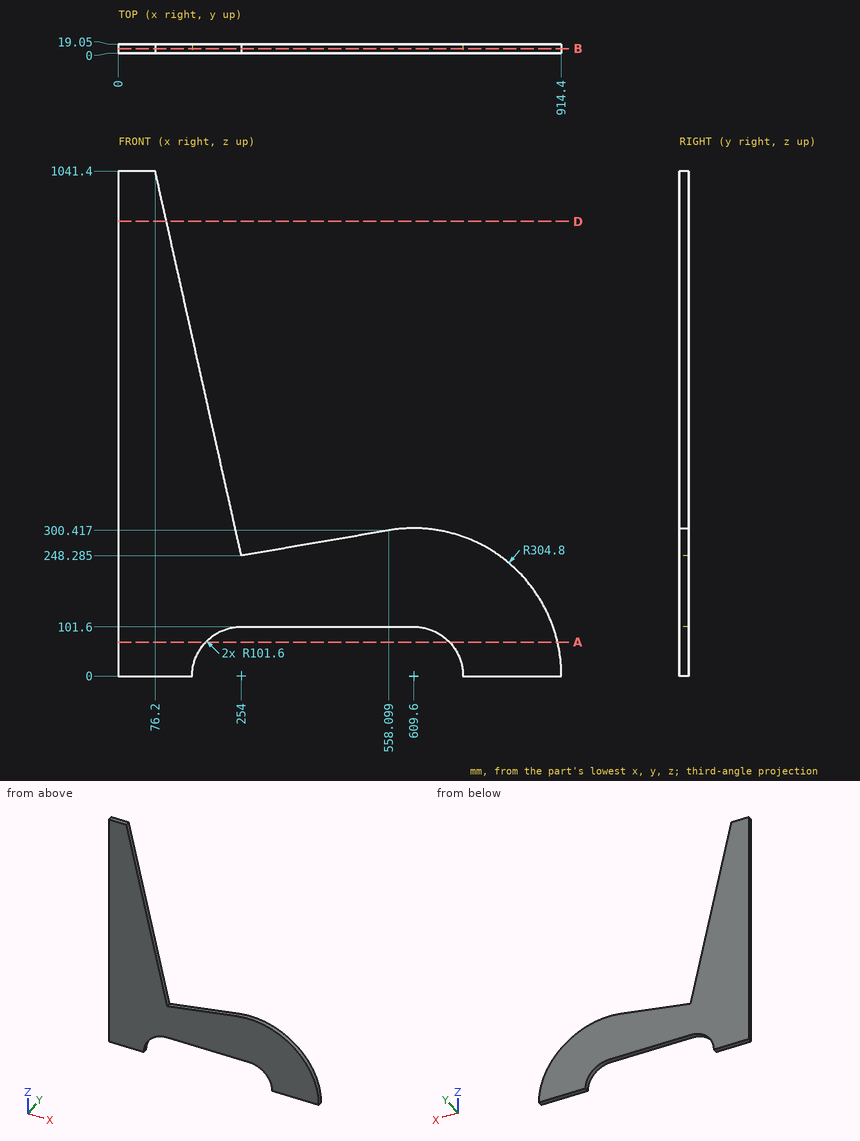
Print and shaded views of the part. All mm, measured from the part's lowest x, y and z. Coordinates: 2 decimals unless noted, no trailing zeros. Order: outer loops, then holes, each group sorted by start corner. A loop starts at its lowest first (then second) coordinate and runs counter-clockwise, first axis right, second up. Notation, with made-up numbers: M 28,-8 L 58,-8 A25 ccw 58,23 Z; hole C 87.5,-30 d9. An arc over 180 degrees is marked long. Write each question's results on one line, items separated by ' | '. Start each with the question number.
Q1. Cut at A-A (z = 70). List the corners of the cut face in (x, y).
Q2. Drill centre lines: probe 1 along X at (y, z) = (7.75, 856.5); probe 2 along X at (y, z) = (16.75, 963.5) (1 decimal); probe 3 along Z at (x, y) = (445, 17.5). Where is each one in solid material? Low to high. Write a range as from..to.
Q3. Cut at D-D (z = 938). List the corners of the cut face in (x, y).
Q4. Flat gauge pins, fed straight in: P1, Ø1.5, axis at y = 16.5, z = 257.5, coming from the +X side (1 decimal); P2, Ø10, axis at y = 4.5, z = 932, coming from the +X side; P3, Ø3, axis at x = 351, y = 11, coming from the +Z side. Where does each tip first touch, or does it go through?
Q5. Cut at B-B (y = 9.75). List the corners of the cut face in (x, z) (1 decimal).
Found:
1) outline: M 0,0 L 180.36,0 L 180.36,19.05 L 0,19.05 Z; M 683.24,0 L 906.25,0 L 906.25,19.05 L 683.24,19.05 Z
2) probe 1: 0..117.65 | probe 2: 0..93.7 | probe 3: 101.6..281.03
3) outline: M 0,0 L 99.38,0 L 99.38,19.05 L 0,19.05 Z
4) P1: x = 773.9 | P2: x = 101.85 | P3: z = 265.17
5) outline: M 0,0 L 152.4,0 A101.6 cw 254,101.6 L 609.6,101.6 A101.6 cw 711.2,0 L 914.4,0 A304.8 ccw 558.1,300.4 L 254,248.3 L 76.2,1041.4 L 0,1041.4 Z
